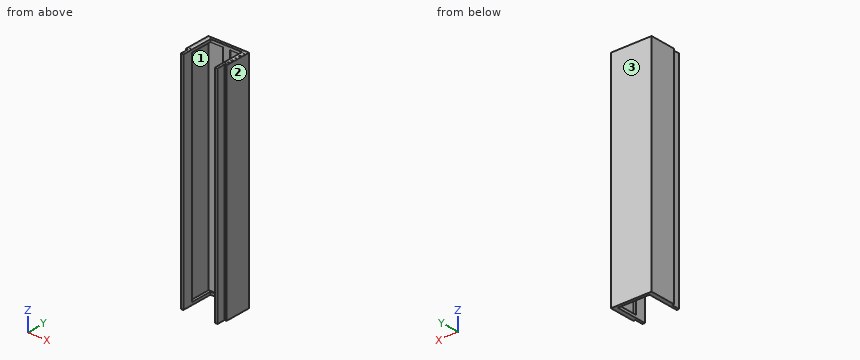
from build123d import *

# Parameters (mm, degrees)
PAD002_DEPTH = 1.45
PAD001_DEPTH = 1.45
PAD_DEPTH    = 120


with BuildPart() as upper_slide:
    # Sketch002 → Pad002 (new body)
    with BuildSketch(Plane(origin=(1.4, -0.5, 118.6), x_dir=(1, 0, 0), z_dir=(0, 0, 1))):
        Polygon((0, -11.7), (-1.4, -11.7), (-1.4, 0.5), (18.6, 0.5), (18.6, -11.7), (17.2, -11.7), (17.2, 0), (0, 0), align=None)
    extrude(amount=PAD002_DEPTH)


with BuildPart() as lower_slide:
    # Sketch001 → Pad001 (new body)
    with BuildSketch(Plane(origin=(1.4, -0.5, 0), x_dir=(1, 0, 0), z_dir=(0, 0, 1))):
        Polygon((0, -11.7), (-1.4, -11.7), (-1.4, 0.5), (18.6, 0.5), (18.6, -11.7), (17.2, -11.7), (17.2, 0), (0, 0), align=None)
    extrude(amount=PAD001_DEPTH)


with BuildPart() as shell:
    # Sketch → Pad (new body)
    with BuildSketch(Plane.XY):
        Polygon((-1, 1), (21, 1), (21, -13.2), (19.9, -13.2), (19.9, -17.7), (18.6, -17.7), (18.6, -12.2), (20, -12.2), (20, 0), (11.9, 0), (11.9, -0.5), (8.1, -0.5), (8.1, 0), (0, 0), (0, -12.2), (1.4, -12.2), (1.4, -17.7), (0.1, -17.7), (0.1, -13.2), (-1, -13.2), align=None)
    extrude(amount=PAD_DEPTH)

    # Fusion: union upper_slide, lower_slide
    add(upper_slide.part)
    add(lower_slide.part)


solid = shell.part
Geometry check sheet. Reference: the model listing, model coordinates, mm. Face numbers are marked on the shaded views. Give positions to 0.01 mm unless a question says otherwise; leave off trailing zeros. Loops run counter-clockwise (first coordinate to the right, second up) from the corner with the lowest first, then second, coordinate; pieces in that order, holes last. Notation, with made-up numbers: (-37, 59.25) -> (21, 59.25) arc R25 ccw to (21, 85.25) -> close; hole circle Ø3 at (67, 2.25). An arc over 180 degrees is marked (long way). Answer in a Markdown table with one row per item. Add a question column.
1) Cross-section at C-C on x = 13.25. Record the boundary of the cut face in (y, z), and give its area (3 significant figures).
2) Cross-section at A-A on y = -16. Record the boundary of the cut face in (x, z).
3) Gauge pin test, flat ends, axial feed: P1, Ø2, axis at x = 3, z = 96.5, coming from the -Y side; P2, Ø8, axis at x = 6.5, z = 15.5, coming from the -Y side; P3, Ø1.3, axis at y = -14.5, z = 80, coming from the +X side. Record the tip position at first contact, or that the pin passes through.
4) Cross-section at D-D on y = -5.5. Record the boundary of the cut face in (x, z).
5) Draft check along Y on the marked faces 1, 2 and 3. Enter one of: pulls with the +Y half, pulls with the -Y half, needs draft (parallel to the pull), parting line crosses it, or undercut.
6) Cross-section at B-B on z = 29. Record the boundary of the cut face in (x, y), and give its area (3 significant figures).
7) Material ranges on probe 1 along X at (y, z) = (-0.25, 63.5); probe 2 along X at (y, z) = (-11.5, 90); probe 3 along X at (y, z) = (-16.5, 83.5), recorded low to high. Write a range as from..to.
Outcome:
| question | item | result |
|---|---|---|
| 1 | outline | (-0.5, 0) -> (1, 0) -> (1, 120) -> (0, 120) -> (0, 120.05) -> (-0.5, 120.05) -> (-0.5, 118.6) -> (0, 118.6) -> (0, 1.45) -> (-0.5, 1.45) -> close |
| 1 | area | 121 mm^2 |
| 2 | outline | (0.1, 0) -> (1.4, 0) -> (1.4, 120) -> (0.1, 120) -> close; (18.6, 0) -> (19.9, 0) -> (19.9, 120) -> (18.6, 120) -> close |
| 3 | P1 | stops at y = 0 |
| 3 | P2 | stops at y = -0.5 |
| 3 | P3 | stops at x = 19.9 |
| 4 | outline | (-1, 0) -> (1.4, 0) -> (1.4, 1.45) -> (0, 1.45) -> (0, 118.6) -> (1.4, 118.6) -> (1.4, 120.05) -> (0, 120.05) -> (0, 120) -> (-1, 120) -> close; (18.6, 0) -> (21, 0) -> (21, 120) -> (20, 120) -> (20, 120.05) -> (18.6, 120.05) -> (18.6, 118.6) -> (20, 118.6) -> (20, 1.45) -> (18.6, 1.45) -> close |
| 5 | face 1 | undercut |
| 5 | face 2 | needs draft |
| 5 | face 3 | pulls with the +Y half |
| 6 | outline | (-1, -13.2) -> (0.1, -13.2) -> (0.1, -17.7) -> (1.4, -17.7) -> (1.4, -12.2) -> (0, -12.2) -> (0, 0) -> (8.1, 0) -> (8.1, -0.5) -> (11.9, -0.5) -> (11.9, 0) -> (20, 0) -> (20, -12.2) -> (18.6, -12.2) -> (18.6, -17.7) -> (19.9, -17.7) -> (19.9, -13.2) -> (21, -13.2) -> (21, 1) -> (-1, 1) -> close |
| 6 | area | 64.8 mm^2 |
| 7 | probe 1 | x = -1..0, 8.1..11.9, 20..21 |
| 7 | probe 2 | x = -1..0, 20..21 |
| 7 | probe 3 | x = 0.1..1.4, 18.6..19.9 |
